```python
from build123d import *

# Parameters (mm, degrees)
PAD_DEPTH       = 24
SKETCH001_R     = 4.3
POCKET_DEPTH    = 34.301
POCKET001_DEPTH = 5
FILLET_R        = 4
FILLET001_R     = 2


with BuildPart() as part:
    # Sketch → Pad (new body)
    with BuildSketch(Plane.YZ):
        with BuildLine():
            ThreePointArc((-16.039015, -13.4), (20.9, 0), (-16.039015, 13.4))
            Line((-61.6, 13.4), (-16.039015, 13.4))
            Line((-61.6, 13.4), (-61.6, 5.4))
            Line((-61.6, 5.4), (-38.2, 5.4))
            Line((-38.2, 5.4), (-38.2, 2))
            Line((-38.2, 2), (-12.744018, 2))
            ThreePointArc((-12.744018, -2), (12.9, 0), (-12.744018, 2))
            Line((-38.2, -2), (-12.744018, -2))
            Line((-38.2, -5.4), (-38.2, -2))
            Line((-61.6, -5.4), (-38.2, -5.4))
            Line((-61.6, -13.4), (-61.6, -5.4))
            Line((-61.6, -13.4), (-16.039015, -13.4))
        make_face()
    extrude(amount=PAD_DEPTH)

    # Sketch001 (on Face5 of Pad) → Pocket (cut, through all)
    with BuildSketch(Plane(origin=(0, 0, 13.4), x_dir=(0, -1, 0), z_dir=(0, 0, 1))):
        with Locations((50.1, 12)):
            Circle(SKETCH001_R)
        with Locations((27.1, 12)):
            Circle(SKETCH001_R)
    extrude(amount=-POCKET_DEPTH, mode=Mode.SUBTRACT)

    # Sketch002 (on Face7 of Pocket) → Pocket001 (cut)
    with BuildSketch(Plane.YX.offset(13.4)):
        Polygon((-43.5, 8.189488), (-43.5, 15.810512), (-50.1, 19.621024), (-56.7, 15.810512), (-56.7, 8.189488), (-50.1, 4.378976), align=None)
        Polygon((-20.5, 8.189488), (-20.5, 15.810512), (-27.1, 19.621024), (-33.7, 15.810512), (-33.7, 8.189488), (-27.1, 4.378976), align=None)
    extrude(amount=-POCKET001_DEPTH, mode=Mode.SUBTRACT)

    # Fillet
    fillet_edges = [part.edges().sort_by_distance(p)[0] for p in [
        (12, -16.039015, -13.4),
        (12, -16.039015, 13.4),
        (0, -61.6, 9.4),
        (24, -61.6, 9.4),
        (0, -61.6, -9.4),
        (24, -61.6, -9.4),
    ]]
    fillet(fillet_edges, radius=FILLET_R)

    # Fillet001
    fillet001_edges = [part.edges().sort_by_distance(p)[0] for p in [
        (0, -37.705757, -13.4),
    ]]
    fillet(fillet001_edges, radius=FILLET001_R)


solid = part.part
```
Geometry: final body of the model. Coordinates: model frame, mm. A direction names the side the tool comes from. Round coordinates to 2 decimals unless told otherwise and drop trailing zeros. Order: outer loops, then holes, each group sorted by start corner. A loop starts at its lowest first (then second) coordinate and runs counter-clockwise, first axis right, second up. Notation, with made-up numbers: (37.25, 62) -> (77.25, 62) arc R29 ccw to (77.25, 92) -> close; hole circle Ø6 at (-27, 11). An arc over 180 degrees is marked (long way). Write each question's results on one line, items separated by ' | '.
Q1. Section query C-C (x = 5.5). Output: boundary loops of the cut face in (y, z), and give its area (3 significant figures).
Response values:
outline: (-61.6, -11.4) arc R2 ccw to (-59.6, -13.4) -> (-52.04, -13.4) -> (-52.04, -8.4) -> (-48.16, -8.4) -> (-48.16, -13.4) -> (-29.04, -13.4) -> (-29.04, -8.4) -> (-25.16, -8.4) -> (-25.16, -13.4) -> (-17.81, -13.4) arc R4 cw to (-14.95, -14.6) arc R20.9 ccw (long way) to (-14.95, 14.6) arc R4 cw to (-17.81, 13.4) -> (-59.6, 13.4) arc R2 ccw to (-61.6, 11.4) -> (-61.6, 5.4) -> (-38.2, 5.4) -> (-38.2, 2) -> (-12.74, 2) arc R12.9 cw (long way) to (-12.74, -2) -> (-38.2, -2) -> (-38.2, -5.4) -> (-61.6, -5.4) -> close | area: 1,590 mm²
Q2. Pull-direction query (X, two-part tool) for faces 1 (the face through (0.57, -37.98, 12.8)), 2 (the face through (12.189, -45.804, 9.456)), 3 (the face through (12.14, -16.24, 13.72)); classes: released by +X, released by -X, zero draft, split by the parting line, or undercut.
Response values:
face 1: released by -X | face 2: undercut | face 3: zero draft
Q3. Pin query (flat end, axial travel): pin 1 Ø1.5 at (x, z) = (13.5, -9.5) entering from +Y; pin 2 Ø1.7 at (x, z) = (14.5, 3) entering from -Y; pin 3 Ø3 at (y, z) = (0.5, -11) entering from +X; pin 4 Ø1.5 at (x, z) = (11, -10.5) entering from +Y. Return the tip coordinate at first contact, or that it passes through.
Response values:
pin 1: y = 18.98 | pin 2: y = -38.2 | pin 3: through | pin 4: y = 18.49
Q4. Section query D-D (x = 12). Count the separate pieces of the cut face and the enclosed holes in it, and give its area (3 significant figures).
Response values:
separate pieces: 5 | enclosed holes: 0 | area: 1,250 mm²
Q5. Access query for faces 4 (the face through (9, -23, -2)), 5 (the face through (16.263, -26.54, -5.155)), 6 (the face through (17.689, -23.754, -10.935)), 7 (the face through (12, -39, -13.4)), 8 (the face through (23.43, -37.43, 12.8)). Directions: +Z, -Z, +X, -X, +Y, -Y. A direction counts if a zero-diameter tool reaches every point of the face in a straight line with its end or side. Return the directions, or none.
Response values:
face 4: +X, -X, -Y | face 5: +Z, -Z | face 6: -Z | face 7: -Z, +X, -X, -Y | face 8: +Z, +X, -Y
Q6. Section query B-B (z = 0). Output: boundary loops of the cut face in (x, y).
Response values:
outline: (0, 12.9) -> (24, 12.9) -> (24, 18.9) arc R2 ccw to (22, 20.9) -> (2, 20.9) arc R2 ccw to (0, 18.9) -> close
Q7. Ray query, line 1 along X through (y, z) = (-27, 4); line 2 along Z through (x, y) = (6.75, -54.5); line 3 along Y through (x, z) = (5.25, -6). Return the intervals inside material, ascending.
Response values:
line 1: 0 to 7.7, 16.3 to 24 | line 2: -13.4 to -5.4, 5.4 to 13.4 | line 3: -61.6 to -11.42, 11.42 to 20.02
Q8. Section query A-A (y = -39). Output: boundary loops of the cut face in (x, z).
Response values:
outline: (0, -11.4) arc R2 ccw to (2, -13.4) -> (22, -13.4) arc R2 ccw to (24, -11.4) -> (24, -5.4) -> (0, -5.4) -> close; (0, 5.4) -> (24, 5.4) -> (24, 11.4) arc R2 ccw to (22, 13.4) -> (2, 13.4) arc R2 ccw to (0, 11.4) -> close
